```python
from build123d import *

# Parameters (mm, degrees)
F1_DEPTH = 6.35


with BuildPart() as f1:
    # F0 (on Front) → F1 (new body, symmetric)
    with BuildSketch(Plane.XZ):
        with BuildLine():
            Line((-39.895691, -12.556188), (-39.895691, -63.356188))
            Line((-39.895691, -63.356188), (4.725324, -63.356188))
            Line((4.725324, -63.356188), (4.725324, -12.556188))
            ThreePointArc((4.725324, -12.556188), (-17.585183, 9.754319), (-39.895691, -12.556188))
        make_face()
        Polygon((0, 90.262515), (-64.81318, 27.438652), (64.81318, 27.438652), align=None)
        with BuildLine():
            Line((-64.81318, 27.438652), (-64.81318, -63.356188))
            Line((-64.81318, -63.356188), (-39.895691, -63.356188))
            Line((-39.895691, -63.356188), (-39.895691, -12.556188))
            ThreePointArc((-39.895691, -12.556188), (-17.585183, 9.754319), (4.725324, -12.556188))
            Line((4.725324, -12.556188), (4.725324, -63.356188))
            Line((4.725324, -63.356188), (64.81318, -63.356188))
            Line((64.81318, -63.356188), (64.81318, 27.438652))
            Line((64.81318, 27.438652), (-64.81318, 27.438652))
        make_face()
    extrude(amount=F1_DEPTH, both=True)


solid = f1.part
```
Verification items for the finished model (mm, model axes). Coordinates: 2 decimals unless noted, no trailing zeros. Write each loop counter-clockwise with the first axis right and the second up, starting at its lowest first coordinate (ties: lowest second). Pieces come first, ordered by that corner, then holes. Notation, with made-up numbers: M 89.25,39.25 L 127.25,39.25 A22 cw 127.25,55.25 Z; hole C 10,-28.5 d4. An arc over 180 degrees is marked long. Answer as a JSON object with one key per item and string values. Group by question number.
(1) Gauge pin test, flat ends, axial feed: pin 1 (3 mm diameter, centred on y = 3, z = 46.5, fed in from +X); pin 2 (1 mm diameter, centred on x = -43.5, y = 0, fed in from +Z); pin 3 (6 mm diameter, centred on y = 1, z = 39.5, fed in from +X). Record the tip position at first contact, or that the pin passes through.
(2) Cross-section at C-C, the plane z = 33.5. Record the cut outline in (x, y), and give its area (3 significant figures).
(3) Cross-section at A-A, the plane y = 3.5. Record the cut outline in (x, z), and give its area (3 significant figures).
(4) Material ranges on line 1 (Z direction, x = 11, y = -2); line 2 (Z direction, x = -16.5, y = -1); line 3 (X direction, y = 3.5, z = 32), recorded low to high.
(5) Cross-section at B-B, the plane x = -8.5. Record the cut outline in (y, z).
Reply:
{
 "1": {"pin 1": "x = 46.7", "pin 2": "z = 48.58", "pin 3": "x = 55.46"},
 "2": {"outline": "M -58.56,-6.35 L 58.56,-6.35 L 58.56,6.35 L -58.56,6.35 Z", "area": "1,490 mm²"},
 "3": {"outline": "M -64.81,-63.36 L 64.81,-63.36 L 64.81,27.44 L 0,90.26 L -64.81,27.44 Z", "area": "15,800 mm²"},
 "4": {"line 1": "-63.36 to 79.6", "line 2": "-63.36 to 74.27", "line 3": "-60.11 to 60.11"},
 "5": {"outline": "M -6.35,-63.36 L 6.35,-63.36 L 6.35,82.02 L -6.35,82.02 Z"}
}
